For this review, use the dimensioned drawing (mm, ordinates from the lowest corner) and the shaded views. A direction names the side the tool comes from. Coordinates: 2 decimals unless noted, no trailing zeros. Order: outer loops, then holes, each group sorted by start corner. A loop starts at its lowest first (then second) coordinate and runs counter-clockwise, first axis right, second up. Notation, with made-up numbers: M 45.25,84.25 L 59.25,84.25 A24 ccw 59.25,123.25 Z; hole C 48.5,-31.75 d3. An arc over 180 degrees is marked long. One line per item, written item: value.
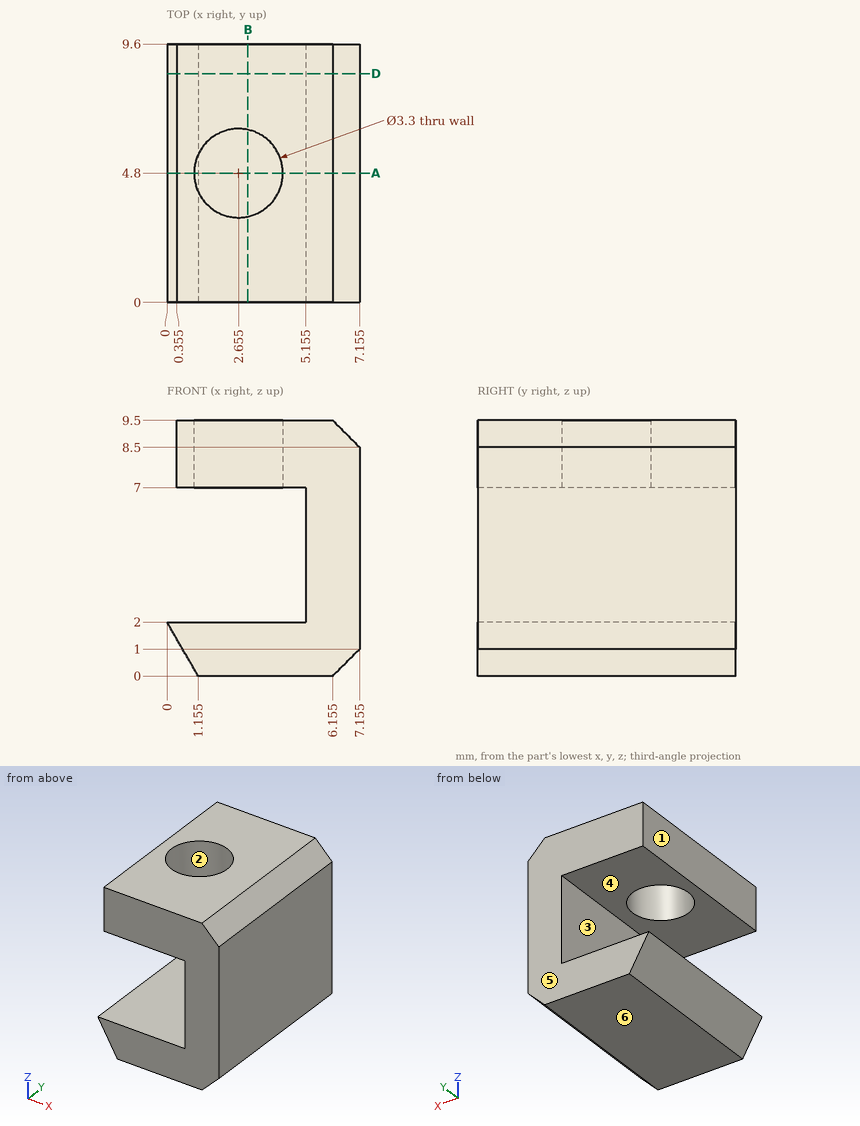
(1) We need section D-D, the plane y = 8.5. State the section outline as (x, z) points (1 decimal).
Geometry results:
outline: M 0,2 L 1.2,0 L 6.2,0 L 7.2,1 L 7.2,8.5 L 6.2,9.5 L 0.4,9.5 L 0.4,7 L 5.2,7 L 5.2,2 Z
(2) Insertion check: pin 1 Ø1.5 at (y, z) = (2.5, 1.5) entering from -X; pin 2 Ø4 at (y, z) = (7, 4.5) entering from -X (1 decimal); pin 3 Ø0.7 at (y, z) = (6, 7.5) entering from -X (1 decimal). Each pin has a flat end and moves straight along its axis. Give the tip position at first contact, or say it passes through.
Geometry results:
pin 1: stops at x = 0
pin 2: stops at x = 5.2
pin 3: stops at x = 0.4
(3) For L1, parallel to Z at x = 1.75, y = 3; L2, parallel to X at y = 3, z = 8.25 (1 decimal); L3, parallel to X at y = 4.75, z = 2.25 (1 decimal), list the stretches that pass through material, from the lowest coordinate up.
Geometry results:
L1: z = 0 to 2, 7 to 9.5
L2: x = 0.4 to 7.2
L3: x = 5.2 to 7.2
(4) Mouldability with a two-part tool opening along Z and no side actions: class the marked faces 4, 5 and 6 as +Z half, -Z half, draft (parallel to the pull), parting line (faces both ways), or undercut.
Geometry results:
face 4: undercut
face 5: draft
face 6: -Z half
(5) We need section B-B, the plane x = 3. State the section outline as (y, z) points.
Geometry results:
outline: M 0,0 L 9.6,0 L 9.6,2 L 0,2 Z; M 0,7 L 3.19,7 L 3.19,9.5 L 0,9.5 Z; M 6.41,7 L 9.6,7 L 9.6,9.5 L 6.41,9.5 Z
(6) Tool access review of the marked faces 1, 2 and 3: name each direction out of +Z, -Z, +X, -X, +Y, -Y from which nothing blocks a thin tool from reaching the whole face with its end or side.
Geometry results:
face 1: +Z, -X, +Y, -Y
face 2: +Z
face 3: -X, +Y, -Y
(7) We need section A-A, the plane y = 4.8. State the section outline as (x, z) points (1 decimal).
Geometry results:
outline: M 0,2 L 1.2,0 L 6.2,0 L 7.2,1 L 7.2,8.5 L 6.2,9.5 L 4.3,9.5 L 4.3,7 L 5.2,7 L 5.2,2 Z; M 0.4,7 L 1,7 L 1,9.5 L 0.4,9.5 Z
